Source: CAD feature listing. Evaluate the final solid. Frame: model axes, mm. Give positions to 0.01 mm unless a question says otherwise; leave off trailing zeros.
from build123d import *

# Parameters (mm, degrees)
F0_W     = 101.6
F0_H     = 2438.4
F1_DEPTH = 101.6
F3_DEPTH = 101.6


with BuildPart() as f1:
    # F0 (on Front) → F1 (new body)
    with BuildSketch(Plane.XZ):
        with Locations((24.5261041723, 1030.4303231494)):
            Rectangle(F0_W, F0_H)
    extrude(amount=F1_DEPTH)

    # F2 (on face) → F3 (cut)
    with BuildSketch(Plane.XZ.offset(101.6)):
        with BuildLine():
            Line((24.5261041723, 1849.5803231494), (24.5261041723, 1887.6803231494))
            ThreePointArc((24.5261041723, 1887.6803231494), (5.4761041723, 1868.6303231494), (24.5261041723, 1849.5803231494))
        make_face()
        with BuildLine():
            ThreePointArc((43.5761041723, 1868.6303231494), (37.9964883539, 1882.100707331), (24.5261041723, 1887.6803231494))
            Line((24.5261041723, 1887.6803231494), (24.5261041723, 1849.5803231494))
            ThreePointArc((24.5261041723, 1849.5803231494), (37.9964883539, 1855.1599389678), (43.5761041723, 1868.6303231494))
        make_face()
        with BuildLine():
            Line((24.5261041723, 1735.2803231494), (24.5261041723, 1773.3803231494))
            ThreePointArc((24.5261041723, 1773.3803231494), (5.4761041723, 1754.3303231494), (24.5261041723, 1735.2803231494))
        make_face()
        with BuildLine():
            ThreePointArc((43.5761041723, 1754.3303231494), (37.9964883539, 1767.800707331), (24.5261041723, 1773.3803231494))
            Line((24.5261041723, 1773.3803231494), (24.5261041723, 1735.2803231494))
            ThreePointArc((24.5261041723, 1735.2803231494), (37.9964883539, 1740.8599389678), (43.5761041723, 1754.3303231494))
        make_face()
        with BuildLine():
            Line((24.5261041723, 1620.9803231494), (24.5261041723, 1659.0803231494))
            ThreePointArc((24.5261041723, 1659.0803231494), (5.4761041723, 1640.0303231494), (24.5261041723, 1620.9803231494))
        make_face()
        with BuildLine():
            ThreePointArc((43.5761041723, 1640.0303231494), (37.9964883539, 1653.500707331), (24.5261041723, 1659.0803231494))
            Line((24.5261041723, 1659.0803231494), (24.5261041723, 1620.9803231494))
            ThreePointArc((24.5261041723, 1620.9803231494), (37.9964883539, 1626.5599389678), (43.5761041723, 1640.0303231494))
        make_face()
        with BuildLine():
            ThreePointArc((24.5261041723, 1544.7803231494), (5.4761041723, 1525.7303231494), (24.5261041723, 1506.6803231494))
            Line((24.5261041723, 1506.6803231494), (24.5261041723, 1544.7803231494))
        make_face()
        with BuildLine():
            Line((24.5261041723, 1430.4803231494), (24.5261041723, 1392.3803231494))
            ThreePointArc((24.5261041723, 1392.3803231494), (37.9964883539, 1397.9599389678), (43.5761041723, 1411.4303231494))
            ThreePointArc((43.5761041723, 1411.4303231494), (37.9964883539, 1424.900707331), (24.5261041723, 1430.4803231494))
        make_face()
        with BuildLine():
            ThreePointArc((24.5261041723, 1430.4803231494), (5.4761041723, 1411.4303231494), (24.5261041723, 1392.3803231494))
            Line((24.5261041723, 1392.3803231494), (24.5261041723, 1430.4803231494))
        make_face()
        with BuildLine():
            Line((24.5261041723, 1544.7803231494), (24.5261041723, 1506.6803231494))
            ThreePointArc((24.5261041723, 1506.6803231494), (37.9964883539, 1512.2599389678), (43.5761041723, 1525.7303231494))
            ThreePointArc((43.5761041723, 1525.7303231494), (37.9964883539, 1539.200707331), (24.5261041723, 1544.7803231494))
        make_face()
        with BuildLine():
            Line((24.5261041723, 1316.1803231494), (24.5261041723, 1278.0803231494))
            ThreePointArc((24.5261041723, 1278.0803231494), (37.9964883539, 1283.6599389678), (43.5761041723, 1297.1303231494))
            ThreePointArc((43.5761041723, 1297.1303231494), (37.9964883539, 1310.600707331), (24.5261041723, 1316.1803231494))
        make_face()
        with BuildLine():
            ThreePointArc((24.5261041723, 1316.1803231494), (5.4761041723, 1297.1303231494), (24.5261041723, 1278.0803231494))
            Line((24.5261041723, 1278.0803231494), (24.5261041723, 1316.1803231494))
        make_face()
        with BuildLine():
            ThreePointArc((24.5261041723, 1201.8803231494), (5.4761041723, 1182.8303231494), (24.5261041723, 1163.7803231494))
            Line((24.5261041723, 1163.7803231494), (24.5261041723, 1201.8803231494))
        make_face()
        with BuildLine():
            Line((24.5261041723, 1201.8803231494), (24.5261041723, 1163.7803231494))
            ThreePointArc((24.5261041723, 1163.7803231494), (37.9964883539, 1169.3599389678), (43.5761041723, 1182.8303231494))
            ThreePointArc((43.5761041723, 1182.8303231494), (37.9964883539, 1196.300707331), (24.5261041723, 1201.8803231494))
        make_face()
        with BuildLine():
            ThreePointArc((43.5761041723, 1068.5303231494), (37.9964883539, 1082.000707331), (24.5261041723, 1087.5803231494))
            Line((24.5261041723, 1087.5803231494), (24.5261041723, 1049.4803231494))
            ThreePointArc((24.5261041723, 1049.4803231494), (37.9964883539, 1055.0599389678), (43.5761041723, 1068.5303231494))
        make_face()
        with BuildLine():
            Line((24.5261041723, 1049.4803231494), (24.5261041723, 1087.5803231494))
            ThreePointArc((24.5261041723, 1087.5803231494), (5.4761041723, 1068.5303231494), (24.5261041723, 1049.4803231494))
        make_face()
        with BuildLine():
            Line((24.5261041723, 935.1803231494), (24.5261041723, 973.2803231494))
            ThreePointArc((24.5261041723, 973.2803231494), (5.4761041723, 954.2303231494), (24.5261041723, 935.1803231494))
        make_face()
        with BuildLine():
            ThreePointArc((43.5761041723, 954.2303231494), (37.9964883539, 967.700707331), (24.5261041723, 973.2803231494))
            Line((24.5261041723, 973.2803231494), (24.5261041723, 935.1803231494))
            ThreePointArc((24.5261041723, 935.1803231494), (37.9964883539, 940.7599389678), (43.5761041723, 954.2303231494))
        make_face()
        with BuildLine():
            ThreePointArc((24.5261041723, 858.9803231494), (5.4761041723, 839.9303231494), (24.5261041723, 820.8803231494))
            Line((24.5261041723, 820.8803231494), (24.5261041723, 858.9803231494))
        make_face()
        with BuildLine():
            Line((24.5261041723, 858.9803231494), (24.5261041723, 820.8803231494))
            ThreePointArc((24.5261041723, 820.8803231494), (37.9964883539, 826.4599389678), (43.5761041723, 839.9303231494))
            ThreePointArc((43.5761041723, 839.9303231494), (37.9964883539, 853.400707331), (24.5261041723, 858.9803231494))
        make_face()
        with BuildLine():
            ThreePointArc((24.5261041723, 744.6803231494), (5.4761041723, 725.6303231494), (24.5261041723, 706.5803231494))
            Line((24.5261041723, 706.5803231494), (24.5261041723, 744.6803231494))
        make_face()
        with BuildLine():
            Line((24.5261041723, 744.6803231494), (24.5261041723, 706.5803231494))
            ThreePointArc((24.5261041723, 706.5803231494), (37.9964883539, 712.1599389678), (43.5761041723, 725.6303231494))
            ThreePointArc((43.5761041723, 725.6303231494), (37.9964883539, 739.100707331), (24.5261041723, 744.6803231494))
        make_face()
        with BuildLine():
            Line((24.5261041723, 592.2803231494), (24.5261041723, 630.3803231494))
            ThreePointArc((24.5261041723, 630.3803231494), (5.4761041723, 611.3303231494), (24.5261041723, 592.2803231494))
        make_face()
        with BuildLine():
            ThreePointArc((43.5761041723, 611.3303231494), (37.9964883539, 624.800707331), (24.5261041723, 630.3803231494))
            Line((24.5261041723, 630.3803231494), (24.5261041723, 592.2803231494))
            ThreePointArc((24.5261041723, 592.2803231494), (37.9964883539, 597.8599389678), (43.5761041723, 611.3303231494))
        make_face()
        with BuildLine():
            ThreePointArc((24.5261041723, 516.0803231494), (5.4761041723, 497.0303231494), (24.5261041723, 477.9803231494))
            Line((24.5261041723, 477.9803231494), (24.5261041723, 516.0803231494))
        make_face()
        with BuildLine():
            Line((24.5261041723, 516.0803231494), (24.5261041723, 477.9803231494))
            ThreePointArc((24.5261041723, 477.9803231494), (37.9964883539, 483.5599389678), (43.5761041723, 497.0303231494))
            ThreePointArc((43.5761041723, 497.0303231494), (37.9964883539, 510.500707331), (24.5261041723, 516.0803231494))
        make_face()
        with BuildLine():
            ThreePointArc((24.5261041723, 401.7803231494), (5.4761041723, 382.7303231494), (24.5261041723, 363.6803231494))
            Line((24.5261041723, 363.6803231494), (24.5261041723, 401.7803231494))
        make_face()
        with BuildLine():
            Line((24.5261041723, 401.7803231494), (24.5261041723, 363.6803231494))
            ThreePointArc((24.5261041723, 363.6803231494), (37.9964883539, 369.2599389678), (43.5761041723, 382.7303231494))
            ThreePointArc((43.5761041723, 382.7303231494), (37.9964883539, 396.200707331), (24.5261041723, 401.7803231494))
        make_face()
        with BuildLine():
            ThreePointArc((24.5261041723, 287.4803231494), (5.4761041723, 268.4303231494), (24.5261041723, 249.3803231494))
            Line((24.5261041723, 249.3803231494), (24.5261041723, 268.4303231494))
            Line((24.5261041723, 268.4303231494), (24.5261041723, 287.4803231494))
        make_face()
        with BuildLine():
            Line((24.5261041723, 268.4303231494), (24.5261041723, 249.3803231494))
            ThreePointArc((24.5261041723, 249.3803231494), (37.9964883539, 254.9599389678), (43.5761041723, 268.4303231494))
            ThreePointArc((43.5761041723, 268.4303231494), (37.9964883539, 281.900707331), (24.5261041723, 287.4803231494))
            Line((24.5261041723, 287.4803231494), (24.5261041723, 268.4303231494))
        make_face()
    extrude(amount=-F3_DEPTH, mode=Mode.SUBTRACT)


solid = f1.part
(1) Section A-A, the plane y = -41.5. Count the separate pieces of the cut face and the enclosed holes in it, plus the area to 3 significant figures.
(2) Line query: line 1 along X through (y, z) = (-71.5, 1429). Output: solid intervals per line, ascending.
(3) Pin query (flat end, axial travel): pin 1 Ø23 at (x, z) = (24.53, 839.93) entering from +Y. Return the tip coordinate at first contact, or that it passes through.
(4) Draft query along Z for faces 1 (the flat face through (24, -101.6, 1047)), 2 (the cylindrical face through (34.77, -51.51, 1198.89)), 3 (the flat face through (24, -50, -188.77)). Return one class per face: +Z half, -Z half, draft (parallel to the pull), parting line (faces both ways), or undercut.
Checks:
1. separate pieces: 1
1. enclosed holes: 15
1. area: 231,000 mm2
2. line 1: x = -26.27 to 17.16, 31.89 to 75.33
3. pin 1: passes through
4. face 1: draft
4. face 2: undercut
4. face 3: -Z half
